```python
from build123d import *

# Parameters (mm, degrees)
MODEL_R             = 1.300000004
MODEL_R_2           = 1.300000002
BOSS_EXTRUDE1_DEPTH = 3


with BuildPart() as part:
    # Model → Boss-Extrude1 (new body)
    with BuildSketch(Plane.XY):
        with BuildLine():
            Line((40.053989941, 38.263739991), (41.750869933, 39.960959983))
            Line((41.750869933, 39.960959983), (45.993869928, 35.718559999))
            Line((45.993869928, 35.718559999), (48.115019916, 37.840109993))
            ThreePointArc((48.115019916, 37.840109993), (49.386777149, 37.499408798), (50.317678177, 38.430465746))
            Line((50.317678177, 38.430465746), (52.154393357, 45.286895639))
            ThreePointArc((52.154393357, 45.286895639), (52.160230302, 46.299486533), (51.669359128, 47.185161347))
            ThreePointArc((51.669359128, 47.185161347), (53.96779664, 53.902048674), (58.141990239, 48.159619035))
            ThreePointArc((58.141990239, 48.159619035), (58.061248273, 47.975250139), (57.99941682, 47.783708953))
            Line((57.99941682, 47.783708953), (54.831453076, 35.957184914))
            ThreePointArc((54.831453076, 35.957184914), (54.831683355, 32.419225016), (56.600919899, 29.355410018))
            Line((56.600919899, 29.355410018), (54.479669903, 27.233960017))
            Line((54.479669903, 27.233960017), (58.722669898, 22.991560033))
            Line((58.722669898, 22.991560033), (57.025689898, 21.294440033))
            Line((57.025689898, 21.294440033), (52.782789911, 25.536740025))
            Line((52.782789911, 25.536740025), (50.661639908, 23.415390031))
            Line((50.661639908, 23.415390031), (42.175739933, 31.899990006))
            Line((42.175739933, 31.899990006), (44.296889928, 34.02144))
            Line((44.296889928, 34.02144), (40.053989941, 38.263739991))
        make_face()
        with Locations((49.388329912, 30.627700012)):
            Circle(MODEL_R, mode=Mode.SUBTRACT)
        with Locations((54.563263872, 49.946565983)):
            Circle(MODEL_R_2, mode=Mode.SUBTRACT)
    extrude(amount=BOSS_EXTRUDE1_DEPTH)


solid = part.part
```
Verification items for the finished model (mm, model axes). A direction names the side the tool comes from. Coordinates: 2 decimals unless noted, no trailing zeros. Loops run counter-clockwise (first coordinate to the right, second up) from the corner with the lowest first, then second, coordinate; pieces in that order, holes last. Notation, with made-up numbers: (-9, 82) - (12, 82) arc R21 ccw to (12, 89) - close; hole circle Ø5 at (69, -23). An arc over 180 degrees is marked (long way). Return JSON: item names as keys, results as strings.
1. Mould release check, pull along X, two halves, no side actions. Record for faces 6 (the flat face through (56.438, 41.953, 1.479)), 7 (the flat face through (46.478, 27.598, 1.479)), 8 (the flat face through (47.04, 36.764, 1.479)): +X half, -X half, draft (parallel to the pull), parting line (faces both ways), or undercut.
Established:
{"face 6": "+X half", "face 7": "-X half", "face 8": "undercut"}
2. Section check C-C, the plane z = 1.5. Record the boundary of the cut face in (x, y).
Established:
{"outline": "(40.05, 38.26) - (44.3, 34.02) - (42.18, 31.9) - (50.66, 23.42) - (52.78, 25.54) - (57.03, 21.29) - (58.72, 22.99) - (54.48, 27.23) - (56.6, 29.36) arc R6.83 cw to (54.83, 35.96) - (58, 47.78) arc R2 cw to (58.14, 48.16) arc R4 ccw (long way) to (51.67, 47.19) arc R2 cw to (52.15, 45.29) - (50.32, 38.43) arc R1.32 cw to (48.12, 37.84) - (45.99, 35.72) - (41.75, 39.96) - close; hole circle Ø2.6 at (49.39, 30.63); hole circle Ø2.6 at (54.56, 49.95)"}
3. Go/stop test with a flat-tipped pin: pin 1 (1 mm diameter, centred on y = 38, z = 1.5, fed in from +X). Record where the tip stops, or that it passes through.
Established:
{"pin 1": "stops at x = 55.51"}
4. Tool access check on faces 1 (the flat face through (43.84, 37.87, 1.48)), 2 (the flat face through (54.93, 23.39, 1.48)), 3 (the flat face through (55.555, 28.31, 1.479)), 4 (the flat face through (43.221, 32.946, 1.479)), 5 (the flat face through (51.223, 41.811, 1.479)). Record the directions out of +Z, -Z, +X, -X, +Y, -Y that give a thin tool (end or side, any length) a straight path to the whole face; none if there is none.
Established:
{"face 1": "+Z, -Z, +Y", "face 2": "+Z, -Z, -Y", "face 3": "+Z, -Z, +X", "face 4": "+Z, -Z, -X", "face 5": "+Z, -Z"}
5. Section check D-D, the plane x = 56.25. Record the boundary of the cut face in (y, z).
Established:
{"outline": "(22.07, 0) - (25.46, 0) - (25.46, 3) - (22.07, 3) - close; (29, 0) - (29.73, 0) - (29.73, 3) - (29, 3) - close; (41.25, 0) - (53.57, 0) - (53.57, 3) - (41.25, 3) - close"}
6. Section check A-A, the plane y = 49.5. Record the boundary of the cut face in (x, z).
Established:
{"outline": "(50.59, 0) - (53.34, 0) - (53.34, 3) - (50.59, 3) - close; (55.78, 0) - (58.54, 0) - (58.54, 3) - (55.78, 3) - close"}
7. Section check B-B, the plane x = 48.5. Record the boundary of the cut face in (y, z).
Established:
{"outline": "(25.58, 0) - (29.68, 0) - (29.68, 3) - (25.58, 3) - close; (31.58, 0) - (37.57, 0) - (37.57, 3) - (31.58, 3) - close"}
8. Thickness scan on L1, parallel to X at y = 50, z = 2.8; L2, parallel to X at y = 24.5, z = 2.95; L3, parallel to Y at x = 48.5, z = 1.45. Record the ranges inside material, lowest first.
Established:
{"L1": "x = 50.56 to 53.26, 55.86 to 58.56", "L2": "x = 49.58 to 51.75, 53.82 to 57.21", "L3": "y = 25.58 to 29.68, 31.58 to 37.57"}
